Can you work these out from the model? Positions are in its coordinate system, mm. Face numbers are marked on the shaded views. Give positions to 0.01 mm unless a question says otherwise; leave off trailing zeros. Order: outer loops, then holes, each group sorted by start corner. A loop starts at its lowest first (then second) coordinate and runs counter-clockwise, first axis right, second up. Notation, with made-up numbers: (30, 87) -> (86, 87) arc R21 cw to (86, 98) -> close; hole circle Ø7 at (-3, 3). An arc over 180 degrees is marked (long way). Answer as CSV lines item,"result".
```python
from build123d import *

# Parameters (mm, degrees)
SKETCH4_R           = 0.85
BOSS_EXTRUDE1_DEPTH = 0.5
FILLET1_R           = 1.826259158
FILLET2_R           = 0.456564789


with BuildPart() as part:
    # Sketch4 → Boss-Extrude1 (new body, symmetric)
    with BuildSketch(Plane.XY):
        with BuildLine():
            Line((-4.356605307, -7.652086329), (-4.179645962, -4.84670606))
            ThreePointArc((-4.179645962, -4.84670606), (-6.422848054, 2.717628201), (0, 7.3))
            Line((0, 7.3), (0, 5.5))
            ThreePointArc((0, 5.5), (-5.499162323, 0.095988235), (-0.191947232, -5.496649549))
            Line((-0.191947232, -5.496649549), (-0.307302772, -8.8))
            ThreePointArc((-0.307302772, -8.8), (-2.401548686, -8.471540527), (-4.356605307, -7.652086329))
        make_face()
        with Locations((-1.950801133, -6.88151398)):
            Circle(SKETCH4_R, mode=Mode.SUBTRACT)
    extrude(amount=BOSS_EXTRUDE1_DEPTH, both=True)

    # Fillet1
    fillet1_edges = [part.edges().sort_by_distance(p)[0] for p in [
        (-4.179645962, -4.84670606, 0),
    ]]
    fillet(fillet1_edges, radius=FILLET1_R)

    # Fillet2
    fillet2_edges = [part.edges().sort_by_distance(p)[0] for p in [
        (-4.356605307, -7.652086329, 0),
    ]]
    fillet(fillet2_edges, radius=FILLET2_R)

    # Mirror1: part across plane


with BuildPart() as part_1:
    add(part.part)
    add(part.part.mirror(Plane(origin=(0, 7.3, 0.5), x_dir=(0, 0, 1), z_dir=(-1, 0, 0))))


solid = part_1.part
```
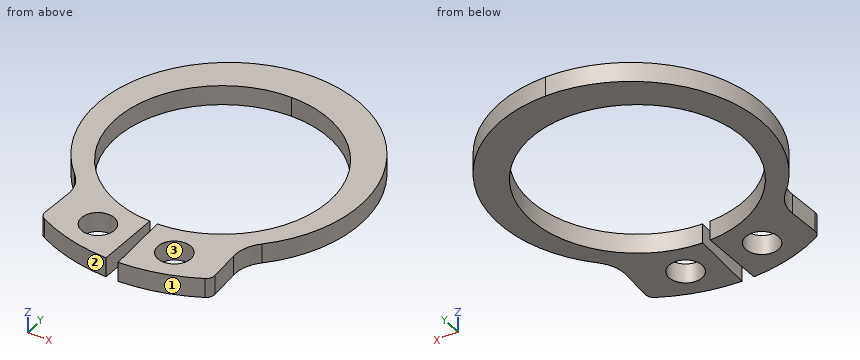
Item 1: Imagine slicing it at C-C, the plane z = -0.15. Please give me the cut outline in (x, y) (3 decimals).
Numbers:
outline,"(-4.775, -4.324) arc R1.826 cw to (-4.236, -5.737) -> (-4.338, -7.362) arc R0.457 ccw to (-4.095, -7.795) arc R8.805 ccw to (-0.307, -8.8) -> (-0.192, -5.497) arc R5.5 cw (long way) to (0.192, -5.497) -> (0.307, -8.8) arc R8.805 ccw to (4.095, -7.795) arc R0.457 ccw to (4.338, -7.362) -> (4.236, -5.737) arc R1.826 cw to (4.775, -4.324) arc R6.792 ccw (long way) to start; hole circle Ø1.7 at (-1.951, -6.882); hole circle Ø1.7 at (1.951, -6.882)"
Item 2: Imagine slicing it at B-B, the plane y = -6.5. Please give me the cut outline in (x, z), then the cut area to 3 significant figures.
Numbers:
outline,"(-4.28, -0.5) -> (-2.71, -0.5) -> (-2.71, 0.5) -> (-4.28, 0.5) -> close; (-1.19, -0.5) -> (-0.23, -0.5) -> (-0.23, 0.5) -> (-1.19, 0.5) -> close; (0.23, -0.5) -> (1.19, -0.5) -> (1.19, 0.5) -> (0.23, 0.5) -> close; (2.71, -0.5) -> (4.28, -0.5) -> (4.28, 0.5) -> (2.71, 0.5) -> close"
area,"5.08 mm²"
Item 3: We'd pull the mould along X, two halves only. Please class the marked faces 1, 2 and 3: released by +X, released by -X, zero draft, split by the parting line, or undercut.
Numbers:
face 1,"released by +X"
face 2,"released by -X"
face 3,"undercut"
Item 4: Please list where these lines run through material, in increasing order: line 1 along X through (y, z) = (-6.25, 0.4); line 2 along Y through (x, z) = (1.25, 0.35); line 3 along X through (y, z) = (-1, -0.05).
Numbers:
line 1,"x = -4.27 to -2.52, -1.38 to -0.22, 0.22 to 1.38, 2.52 to 4.27"
line 2,"y = -8.72 to -7.36, -6.4 to -5.36, 5.36 to 7.18"
line 3,"x = -6.62 to -5.41, 5.41 to 6.62"
Item 5: Imagine slicing it at A-A, the plane x = 2. Please give me the cut outline in (y, z).
Numbers:
outline,"(-8.58, -0.5) -> (-7.73, -0.5) -> (-7.73, 0.5) -> (-8.58, 0.5) -> close; (-6.03, -0.5) -> (-5.12, -0.5) -> (-5.12, 0.5) -> (-6.03, 0.5) -> close; (5.12, -0.5) -> (7, -0.5) -> (7, 0.5) -> (5.12, 0.5) -> close"
Item 6: Imagine slicing it at D-D, the plane x = 0.5. Please give me the cut outline in (y, z), then the cut area to 3 significant figures.
Numbers:
outline,"(-8.79, -0.5) -> (-5.48, -0.5) -> (-5.48, 0.5) -> (-8.79, 0.5) -> close; (5.48, -0.5) -> (7.28, -0.5) -> (7.28, 0.5) -> (5.48, 0.5) -> close"
area,"5.12 mm²"
